Can you work these out from the drawing? Everything is in mm from the part's minimum corner. Give positions to 0.01 mm unless a question says otherwise; leave off trailing zeros. Order: outer loops, then holes, each group sorted by start corner. A loop starts at its lowest first (then second) coordinate and runs counter-clockwise, first axis right, second up. Notation, with made-up numbers: (40, 5.25) - (94, 5.25) arc R12 cw to (94, 23.25) - close; hole circle Ø1 at (20.5, 46.5). An arc over 180 degrees is marked (long way). Write each question's results on one line, items separated by ' | '. Start each with the question number.
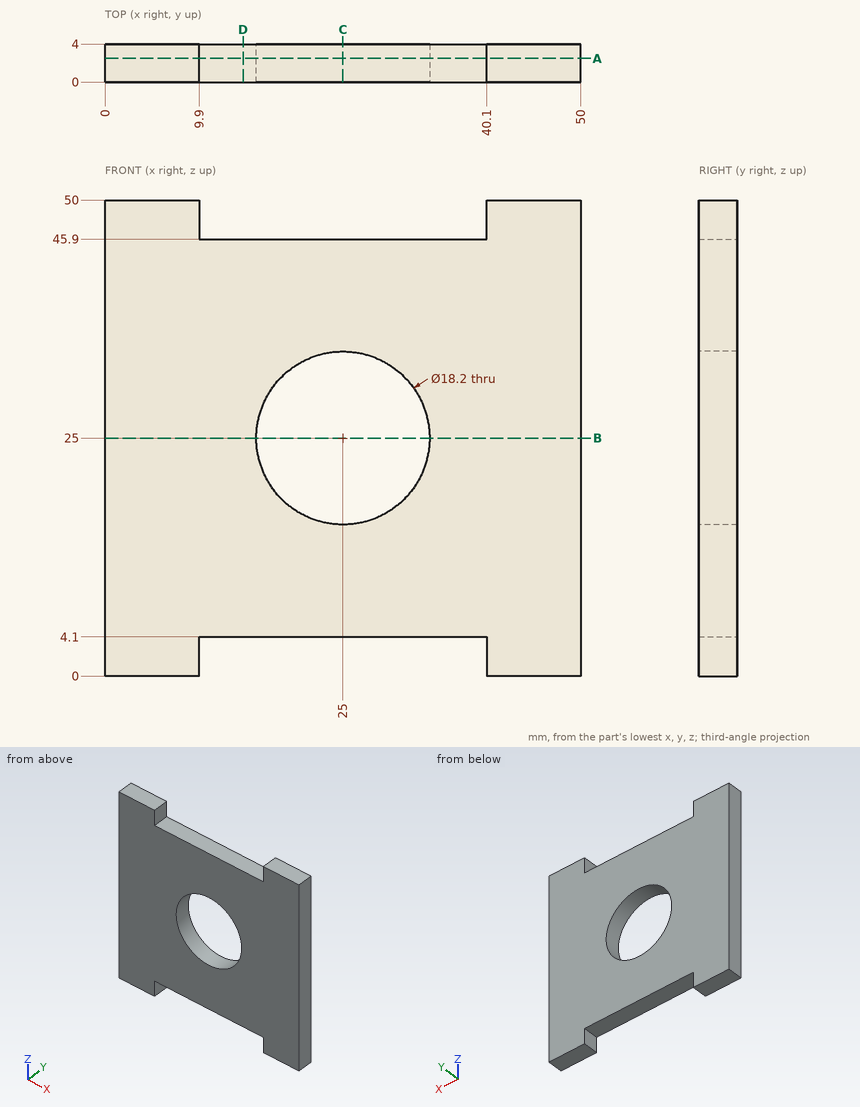
Q1. Will these pins go through, and if not, where does the flat tip stop? P1, Ø1.5, axis at x = 34, y = 0.5, coming from the -Z side; P2, Ø2, axis at x = 31, y = 3, coming from the +Z side.
Q2. If we section it at B-B (z = 25): Please give me the cut outline in (x, y).
Q3. If we section it at A-A (y = 2.5): Please give me the cut outline in (x, z), plus the area to 3 significant figures.
Q4. If we section it at C-C (x = 25): Please give me the cut outline in (y, z).
Q5. If we section it at D-D (x = 14.5): Please give me the cut outline in (y, z).
Q6. If I drill on probe 1 along Z at (x, y) = (25, 2.45); probe 2 along Z at (x, y) = (18.5, 2); probe 3 along X at (y, z) = (1, 2), over which ranges is the centre line in solid material (lowest first)? Write a range as from..to.
Findings below:
1) P1: stops at z = 4.1 | P2: stops at z = 45.9
2) outline: (0, 0) - (15.9, 0) - (15.9, 4) - (0, 4) - close; (34.1, 0) - (50, 0) - (50, 4) - (34.1, 4) - close
3) outline: (0, 0) - (9.9, 0) - (9.9, 4.1) - (40.1, 4.1) - (40.1, 0) - (50, 0) - (50, 50) - (40.1, 50) - (40.1, 45.9) - (9.9, 45.9) - (9.9, 50) - (0, 50) - close; hole circle Ø18.2 at (25, 25) | area: 1,990 mm2
4) outline: (0, 4.1) - (4, 4.1) - (4, 15.9) - (0, 15.9) - close; (0, 34.1) - (4, 34.1) - (4, 45.9) - (0, 45.9) - close
5) outline: (0, 4.1) - (4, 4.1) - (4, 45.9) - (0, 45.9) - close
6) probe 1: z = 4.1..15.9, 34.1..45.9 | probe 2: z = 4.1..18.63, 31.37..45.9 | probe 3: x = 0..9.9, 40.1..50
